Model file for the job. Use its own axes, mm. Face numbers are marked on the shaded views. A direction names the side the tool comes from. Coordinates: 2 decimals unless noted, no trailing zeros. Order: outer loops, then holes, each group sorted by start corner. A loop starts at its lowest first (then second) coordinate and runs counter-clockwise, first axis right, second up. Notation, with made-up numbers: (-5, 23) -> (17, 23) arc R21 ccw to (17, 32) -> close; hole circle Ø3 at (15, 85). An arc over 180 degrees is marked (long way). Use CSV: the item, a comma, the result in double quotes. Start each with the question number.
(1) Probe L1, parallel to Y at x = 0, z = 2.05; L2, parallel to Z at x = 16, y = 3; L3, parallel to Z at x = 13.5, y = 4. List the from-to ranges inside material, lowest first.
(2) Cut at B-B on y = 9.5. Write the cut outline in (x, z), plus the area to 3 significant figures.
(3) Tool access for the marked faces 1, 2 and 3: list every direction of +Z, -Z, +X, -X, +Y, -Y with a clear straight run to the whole face (end or side of a thin tool).
(4) Pin check, flat tips, straight feed: pin 1 Ø1.9 at (x, y) = (0, 9.5) entering from +Z; pin 2 Ø4 at (x, y) = (3.5, 8.5) entering from -Z; pin 3 Ø2.5 at (y, z) = (9.5, 1.5) entering from +X; pin 4 Ø3 at (y, z) = (4.5, 6.5) entering from +X. Stop position of each tip, or through.
(5) Cut at A-A on x = 15.6. Write the cut outline in (y, z).
(6) Cut at C-C on x = 2.25. Write the cut outline in (y, z), plus the area to 3 significant figures.
(7) Cut at D-D on y = 3. Write the cut outline in (x, z).
(8) Pull direction Z, two halves, no side cores. Call the marked faces 4, 5 and 6: pulls with the +Z half, pulls with the -Z half, needs draft (parallel to the pull), parting line crosses it, or undercut.
```python
from build123d import *

# Parameters (mm, degrees)
SKETCH_1_W          = 6
SKETCH_1_H          = 13
SKETCH_1_R          = 1.6
EXTRUDE_1_DEPTH     = 3
SKETCH_3_W          = 21.2
SKETCH_3_H          = 7
EXTRUDE_3_DEPTH     = 13
SKETCH_4_W          = 10.937812939
SKETCH_4_H          = 3.6
CUT_EXTRUDE_1_DEPTH = 13.2
SKETCH_6_R          = 1
EXTRUDE_4_DEPTH     = 2
CHAMFER_1_SIZE      = 0.2


with BuildPart() as part:
    # 草图1 → 拉伸1 (new body)
    with BuildSketch(Plane.XY):
        with Locations((0, 6)):
            Rectangle(SKETCH_1_W, SKETCH_1_H)
        with Locations((0, 9.5)):
            Circle(SKETCH_1_R, mode=Mode.SUBTRACT)
    extrude(amount=EXTRUDE_1_DEPTH)

    # 草图3 → 拉伸3 (add)
    with BuildSketch(Plane(origin=(0, 0, 0), x_dir=(-1, 0, 0), z_dir=(0, 0, -1))):
        with Locations((-7.6, 3)):
            Rectangle(SKETCH_3_W, SKETCH_3_H)
    extrude(amount=-EXTRUDE_3_DEPTH)

    # 草图4 → 切除-拉伸1 (cut)
    with BuildSketch(Plane(origin=(0, 6.5, 0), x_dir=(-1, 0, 0), z_dir=(0, 1, 0))):
        with Locations((-17.068906469, 6.5)):
            Rectangle(SKETCH_4_W, SKETCH_4_H)
    extrude(amount=-CUT_EXTRUDE_1_DEPTH, mode=Mode.SUBTRACT)

    # 草图6 → 拉伸4 (add)
    with BuildSketch(Plane(origin=(0, 0, 0), x_dir=(-1, 0, 0), z_dir=(0, 0, -1))):
        with Locations(Location((-15.6, 3, 0), (0, 0, 180))):
            Circle(SKETCH_6_R)
    extrude(amount=EXTRUDE_4_DEPTH)

    # 倒角1
    chamfer_1_edges = [part.edges().sort_by_distance(p)[0] for p in [
        (14.6, 3, -2),
    ]]
    chamfer(chamfer_1_edges, length=CHAMFER_1_SIZE)


solid = part.part
```
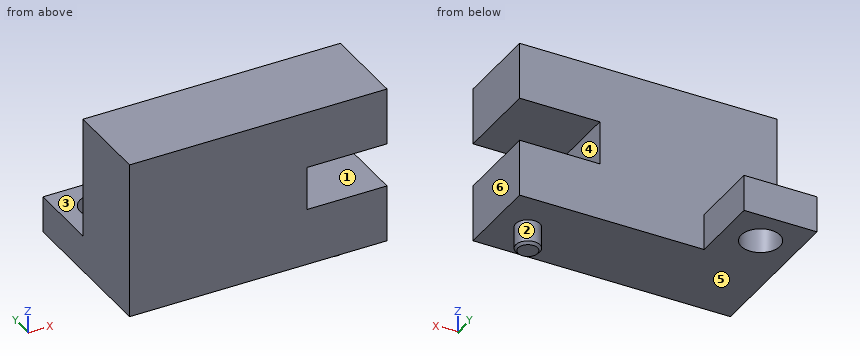
Outcome:
1,L1,"-0.5 to 7.9, 11.1 to 12.5"
1,L2,"-2 to 4.7, 8.3 to 13"
1,L3,"0 to 4.7, 8.3 to 13"
2,outline,"(-3, 0) -> (-1.6, 0) -> (-1.6, 3) -> (-3, 3) -> close; (1.6, 0) -> (3, 0) -> (3, 3) -> (1.6, 3) -> close"
2,area,"8.40 mm2"
3,face 1,"+X, +Y, -Y"
3,face 2,"-Z"
3,face 3,"+Z, +X, -X, +Y"
4,pin 1,"through"
4,pin 2,"z = 0"
4,pin 3,"x = 3"
4,pin 4,"x = 11.6"
5,outline,"(-0.5, 0) -> (2, 0) -> (2, -1.8) -> (2.2, -2) -> (3.8, -2) -> (4, -1.8) -> (4, 0) -> (6.5, 0) -> (6.5, 4.7) -> (-0.5, 4.7) -> close; (-0.5, 8.3) -> (6.5, 8.3) -> (6.5, 13) -> (-0.5, 13) -> close"
6,outline,"(-0.5, 0) -> (12.5, 0) -> (12.5, 3) -> (6.5, 3) -> (6.5, 13) -> (-0.5, 13) -> close"
6,area,"109 mm2"
7,outline,"(-3, 0) -> (14.6, 0) -> (14.6, -1.8) -> (14.8, -2) -> (16.4, -2) -> (16.6, -1.8) -> (16.6, 0) -> (18.2, 0) -> (18.2, 4.7) -> (11.6, 4.7) -> (11.6, 8.3) -> (18.2, 8.3) -> (18.2, 13) -> (-3, 13) -> close"
8,face 4,"undercut"
8,face 5,"pulls with the -Z half"
8,face 6,"needs draft"
